Design review of the part built by this model. Coordinates are the model's own, in mm. A direction names the side the tool comes from. Round coordinates to 2 decimals unless told otherwise and drop trailing zeros. Loops run counter-clockwise (first coordinate to the right, second up) from the corner with the lowest first, then second, coordinate; pieces in that order, holes last. Notation, with made-up numbers: (-1.5, -19.5) -> (17.5, -19.5) arc R19 ccw to (17.5, 0.5) -> close; hole circle Ø1 at (15.25, -34). An arc over 180 degrees is marked (long way). Answer as CSV lines item,"result". Start each with the question number.
(1) Draft analysis for pull direction Y (two halves, no side actions). For faces 1 (the face through (1, 0, 10)), 2 (the face through (36.07, 0.18, -7.46)), 3 (the face through (0, -50.234, 0)), state which applies: +Y half, -Y half, draft (parallel to the pull), parting line (faces both ways), or undercut.
(2) To check wall thickness, follow line 1 (Z direction, x = -8, y = -39.5); line 2 (Z direction, x = 27, y = -8); line 3 (Y direction, x = -1.5, z = -3). State the ranges of each line that lie inside material, in increasing order. Write a range as from..to.
(3) Take a section at B-B, the plane z = -7.5. Write out the cut boundary in (x, y).
(4) Take a section at A-A, the plane y = -33. Write out the cut boundary in (x, z), and give its area (3 significant figures).
(5) Take a section at D-D, the plane z = -3.5. Write out the cut boundary in (x, y).
(6) Take a section at C-C, the plane y = 0. Write out the cut boundary in (x, z), and give its area (3 significant figures).
(7) Machinability: for faces 4 (the face through (-1, 0, 5)), 5 (the face through (0, -15.599, 0)), 6 (the face through (1, 0, -10)), 7 (the face through (0, -29, -20)), which of the approach directions +Z, -Z, +X, -X, +Y, -Y give a long, thin tool a straight path to every point of the face, cutting with its end or side? Answer none if there is none.
(8) For P1, Ø9, axis at x = 25.24, y = 0, coming from the +Z side; P2, Ø13, axis at x = 3.5, y = 0.5, coming from the +Z side; P3, Ø12, axis at y = -29.5, z = 9, coming from the -X side; P4, Ø18, axis at x = -15, y = -3, coming from the -Z side, all flat-tipped, find the tip position at first contact; note any pin that passes through.
from build123d import *

# Parameters (mm, degrees)
BOSS_EXTRUDE1_DEPTH = 10
SKETCH3_W           = 68.02674373
SKETCH3_H           = 42.022590527
BOSS_EXTRUDE2_DEPTH = 20
SKETCH4_W           = 25
SKETCH4_H           = 28
CUT_EXTRUDE1_DEPTH  = 71.084609616
SKETCH5_R           = 5.067107297
CUT_EXTRUDE2_DEPTH  = 31
SKETCH6_W           = 166.597833244
SKETCH6_H           = 42.962518472
CUT_EXTRUDE3_DEPTH  = 5


with BuildPart() as part:
    # Sketch1 → Boss-Extrude1 (new body, symmetric)
    with BuildSketch(Plane.XY):
        with BuildLine():
            Line((-27.860019642, 8.21121811), (27.860019642, 8.21121811))
            ThreePointArc((27.860019642, 8.21121811), (36.071237751, 0), (27.860019642, -8.21121811))
            Line((27.860019642, -8.21121811), (-27.860019642, -8.21121811))
            ThreePointArc((-27.860019642, -8.21121811), (-36.071237751, 0), (-27.860019642, 8.21121811))
        make_face()
    extrude(amount=BOSS_EXTRUDE1_DEPTH, both=True)

    # Sketch3 → Boss-Extrude2 (add, symmetric)
    with BuildSketch(Plane.XY):
        with Locations((0, -29.222513374)):
            Rectangle(SKETCH3_W, SKETCH3_H)
    extrude(amount=BOSS_EXTRUDE2_DEPTH, both=True)

    # Sketch4 → Cut-Extrude1 (cut, through all)
    with BuildSketch(Plane(origin=(34.013371865, 0, 0), x_dir=(0, 0, -1), z_dir=(1, 0, 0))):
        with Locations((0, -29.598628357)):
            Rectangle(SKETCH4_W, SKETCH4_H)
    extrude(amount=-CUT_EXTRUDE1_DEPTH, mode=Mode.SUBTRACT)

    # Sketch5 → Cut-Extrude2 (cut, through all)
    with BuildSketch(Plane.XY.offset(10)):
        with Locations((-25.241020996, 0)):
            Circle(SKETCH5_R)
        with Locations((25.241020996, 0)):
            Circle(SKETCH5_R)
    extrude(amount=-CUT_EXTRUDE2_DEPTH, mode=Mode.SUBTRACT)

    # Sketch6 → Cut-Extrude3 (cut, symmetric)
    with BuildSketch(Plane.XY):
        with Locations((0.75044069, 13.270041126)):
            Rectangle(SKETCH6_W, SKETCH6_H)
    extrude(amount=CUT_EXTRUDE3_DEPTH, both=True, mode=Mode.SUBTRACT)


solid = part.part
The answers:
1,face 1,"draft"
1,face 2,"undercut"
1,face 3,"-Y half"
2,line 1,"-20..-12.5, 12.5..20"
2,line 2,"-10..-5, 5..10"
2,line 3,"-50.23..-43.6, -15.6..-8.21"
3,outline,"(-34.01, -50.23) -> (34.01, -50.23) -> (34.01, -43.6) -> (-34.01, -43.6) -> close; (-34.01, -15.6) -> (34.01, -15.6) -> (34.01, -8.21) -> (27.86, -8.21) arc R8.21 ccw to (27.86, 8.21) -> (-27.86, 8.21) arc R8.21 ccw to (-27.86, -8.21) -> (-34.01, -8.21) -> close; hole circle Ø10.13 at (-25.24, 0); hole circle Ø10.13 at (25.24, 0)"
4,outline,"(-34.01, -20) -> (34.01, -20) -> (34.01, -12.5) -> (-34.01, -12.5) -> close; (-34.01, 12.5) -> (34.01, 12.5) -> (34.01, 20) -> (-34.01, 20) -> close"
4,area,"1,020 mm²"
5,outline,"(-34.01, -50.23) -> (34.01, -50.23) -> (34.01, -43.6) -> (-34.01, -43.6) -> close; (-34.01, -15.6) -> (34.01, -15.6) -> (34.01, -8.21) -> (-34.01, -8.21) -> close"
6,outline,"(-36.07, -10) -> (-30.31, -10) -> (-30.31, -5) -> (-36.07, -5) -> close; (-36.07, 5) -> (-30.31, 5) -> (-30.31, 10) -> (-36.07, 10) -> close; (-20.17, -10) -> (20.17, -10) -> (20.17, -5) -> (-20.17, -5) -> close; (-20.17, 5) -> (20.17, 5) -> (20.17, 10) -> (-20.17, 10) -> close; (30.31, -10) -> (36.07, -10) -> (36.07, -5) -> (30.31, -5) -> close; (30.31, 5) -> (36.07, 5) -> (36.07, 10) -> (30.31, 10) -> close"
6,area,"519 mm²"
7,face 4,"+X, -X, +Y"
7,face 5,"+X, -X"
7,face 6,"-Z, +X, -X, +Y"
7,face 7,"-Z, +X, -X, +Y, -Y"
8,P1,"through"
8,P2,"z = 10"
8,P3,"x = -34.01"
8,P4,"z = -20"
